```python
from build123d import *

# Parameters (mm, degrees)
BOSS_EXTRUDE1_DEPTH     = 3.175
CUT_EXTRUDE1_DEPTH      = 65.189801711
CUT_EXTRUDE1_DEPTH_BACK = 65.189801711
SKETCH3_R               = 1.35
SKETCH3_R_2             = 2.1
SKETCH3_W               = 15
SKETCH3_H               = 7
SKETCH3_W_2             = 25
SKETCH3_H_2             = 11
SKETCH5_W               = 6
SKETCH5_H               = 4.4
CUT_EXTRUDE2_DEPTH      = 65.189801711


with BuildPart() as part:
    # Sketch2 → Boss-Extrude1 (new body)
    with BuildSketch(Plane(origin=(0, 0, 0), x_dir=(1, 0, 0), z_dir=(0, 1, 0))):
        with BuildLine():
            Line((48, 42.5), (-48, 42.5))
            Line((-48, 42.5), (-48, -10.75))
            add(Edge.make_bspline(
                [(-48, -10.75), (-48, -53.083333333), (48, -53.083333333), (48, -10.75)],
                knots=[0, 0, 0, 0, 1, 1, 1, 1], degree=3))
            Line((48, -10.75), (48, 42.5))
        make_face()
    extrude(amount=BOSS_EXTRUDE1_DEPTH)

    # Sketch3 → Cut-Extrude1 (cut, two sides: drawn at the far end of the back side and taken through both)
    with BuildSketch(Plane(origin=(0, 3.175, 0), x_dir=(1, 0, 0), z_dir=(0, 1, 0)).offset(-CUT_EXTRUDE1_DEPTH_BACK)):
        with Locations(Location((-30, 19.5, 0), (0, 0, 270))):
            Circle(SKETCH3_R)
        with Locations(Location((-30, -25.5, 0), (0, 0, 270))):
            Circle(SKETCH3_R)
        with Locations(Location((30, -25.5, 0), (0, 0, 90))):
            Circle(SKETCH3_R)
        with Locations(Location((30, 19.5, 0), (0, 0, 90))):
            Circle(SKETCH3_R)
        with Locations(Location((-29, 4.881263298, 0), (0, 0, 270))):
            Circle(SKETCH3_R_2)
        with Locations(Location((-29, -18.118736702, 0), (0, 0, 270))):
            Circle(SKETCH3_R_2)
        with Locations(Location((29, -18.118736702, 0), (0, 0, 90))):
            Circle(SKETCH3_R_2)
        with Locations(Location((29, 4.881263298, 0), (0, 0, 90))):
            Circle(SKETCH3_R_2)
        with Locations((0, 34.265048758)):
            Rectangle(SKETCH3_W, SKETCH3_H)
        with Locations((-11.5, -18.118736702)):
            Rectangle(SKETCH3_W_2, SKETCH3_H_2)
    extrude(amount=CUT_EXTRUDE1_DEPTH + CUT_EXTRUDE1_DEPTH_BACK, mode=Mode.SUBTRACT)

    # Sketch5 → Cut-Extrude2 (cut, through all)
    with BuildSketch(Plane(origin=(0, 3.175, 0), x_dir=(1, 0, 0), z_dir=(0, 1, 0))):
        with Locations((24.051144599, 40.3)):
            Rectangle(SKETCH5_W, SKETCH5_H)
        with Locations((-23.948855401, 40.3)):
            Rectangle(SKETCH5_W, SKETCH5_H)
    extrude(amount=-CUT_EXTRUDE2_DEPTH, mode=Mode.SUBTRACT)


solid = part.part
```
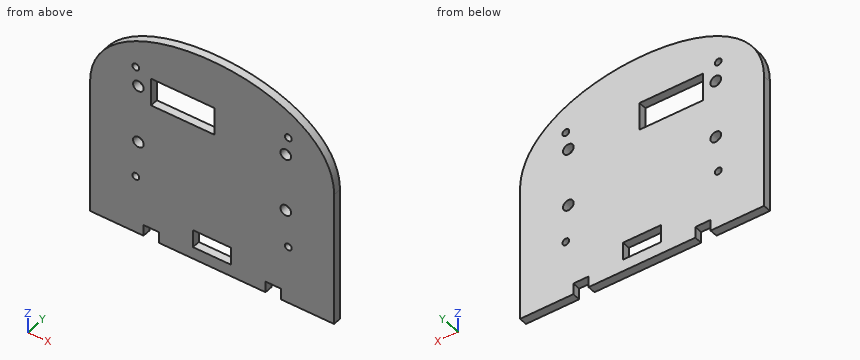
Design review of the part built by this model. Coordinates are the model's own, in mm. Give positions to 0.01 mm unless a question says otherwise; leave off trailing zeros. Loops run counter-clockwise (first coordinate to the right, second up) from the corner with the lowest first, then second, coordinate; pieces in that order, holes last. Notation, with made-up numbers: (-13, -29.75) -> (6, -29.75) arc R17 cw to (6, -14.75) -> close; hole circle Ø5 at (89, -4). An arc over 180 degrees is marked (long way). Write each question's results on one line, items separated by ' | '.
Q1. Take a section at C-C, the plane z = -4. Write out the cut boundary in (x, y) (3 decimals), plus the area to 3 significant figures.
Reply:
outline: (-48, 0) -> (-30.906, 0) -> (-30.906, 3.175) -> (-48, 3.175) -> close; (-27.094, 0) -> (27.094, 0) -> (27.094, 3.175) -> (-27.094, 3.175) -> close; (30.906, 0) -> (48, 0) -> (48, 3.175) -> (30.906, 3.175) -> close | area: 281 mm²
Q2. Take a section at B-B, the plane y = 1.2. Give the number of separate pieces and of enclosed holes in the cut face, plus the area to 3 significant figures.
Reply:
separate pieces: 1 | enclosed holes: 10 | area: 7,040 mm²
Q3. Wall thickness on L1, parallel to X at y = 1, z = 25.5; L2, parallel to Z at x = -30, y = 1; L3, parallel to Z at x = -29, y = 0.9: over which ranges is each line inside the solid? List them lowest first.
Reply:
L1: x = -43.28 to -31.35, -28.65 to 28.65, 31.35 to 43.28 | L2: z = -42.5 to -20.85, -18.15 to -6.73, -3.03 to 16.27, 19.97 to 24.15, 26.85 to 36.18 | L3: z = -42.5 to -20.41, -18.59 to -6.98, -2.78 to 16.02, 20.22 to 24.59, 26.41 to 36.65
Q4. For pin 1 Ø1.6 at (x, y) = (-24.5, 1.5) entering from -Z; pin 2 Ø1.6 at (x, z) = (-30, 25.5) entering from +Y; pin 3 Ø1 at (y, z) = (1, 18.5) entering from -X; pin 4 Ø1 at (x, y) = (-1.5, 1) entering from +Z, all flat-tipped, find the tip position at first contact; note any pin that passes through.
Reply:
pin 1: stops at z = -38.1 | pin 2: passes through | pin 3: stops at x = -46.98 | pin 4: stops at z = 42.49
Q5. Take a section at A-A, the plane z = -19.5. Write out the cut boundary in (x, y) (3 decimals).
Reply:
outline: (-48, 0) -> (-31.35, 0) -> (-31.35, 3.175) -> (-48, 3.175) -> close; (-28.65, 0) -> (28.65, 0) -> (28.65, 3.175) -> (-28.65, 3.175) -> close; (31.35, 0) -> (48, 0) -> (48, 3.175) -> (31.35, 3.175) -> close
